Input: part model. Units: mm. Frame: model coordinates. Face numbers are marked on the shaded views. Round coordinates to 2 decimals unless told otherwise and drop trailing zeros. Loops run counter-clockwise (first coordinate to the right, second up) from the corner with the lowest first, then second, coordinate; pieces in that order, holes last. Notation, with made-up numbers: (15.5, -2.75) -> (65.5, -2.75) arc R28 ccw to (65.5, 16.25) -> close; hole circle Ø6 at (-27.75, 57). An arc over 180 degrees is marked (long way). One line per question, with ' | ' between items. Start each with the question number.
Q1. Material intervals for L1, parallel to Y at x = 30, z = 18; L2, parallel to Y at x = 28.25, z = 14.5; L3, parallel to Z at x = 38.75, y = -10.5, sorted ascending.
Q2. Contact query for flat-ended pins moving along their axis: P1, Ø5, axis at x = 39, y = 26, coming from the +Z side; P2, Ø3, axis at x = 28.5, y = 13.5, coming from the +Z side; P3, Ø8, axis at x = 28.5, z = 25.5, coming from the -Y side. Output: stop coordinate, or through.
Q3. Mould query, pull axis Y, two halves, no side actions, for the marked faces 1, 2 and 3. Classes: pulls with the +Y half, pulls with the -Y half, needs draft (parallel to the pull), parting line crosses it, or undercut.
Q4. Cut plane A-A on x = 46.75. Return loops of the section in (y, z).
Q5. Cut plane C-C on x = 36.75. Return loops of the section in (y, z).
Q6. Cut plane B-B on y = 0. Return loops of the section in (x, z).
from build123d import *

# Parameters (mm, degrees)
SKETCH001_W      = 178.926751
SKETCH001_H      = 164.552085
PAD_DEPTH        = 25
REVOLUTION_ANGLE = 180


with BuildPart() as pad:
    # Sketch001 → Pad (new body)
    with BuildSketch(Plane.YZ):
        with Locations((1.16814, -0.450252)):
            Rectangle(SKETCH001_W, SKETCH001_H)
    extrude(amount=PAD_DEPTH)


with BuildPart() as cut:
    # Sketch → Revolution (revolve)
    with BuildSketch(Plane.XY):
        Polygon((0, 25), (0, 75), (50, 25), align=None)
    revolve(axis=Axis((0, 0, 0), (1, 0, 0)), revolution_arc=REVOLUTION_ANGLE)

    # Cut: cut Pad
    add(pad.part, mode=Mode.SUBTRACT)


solid = cut.part
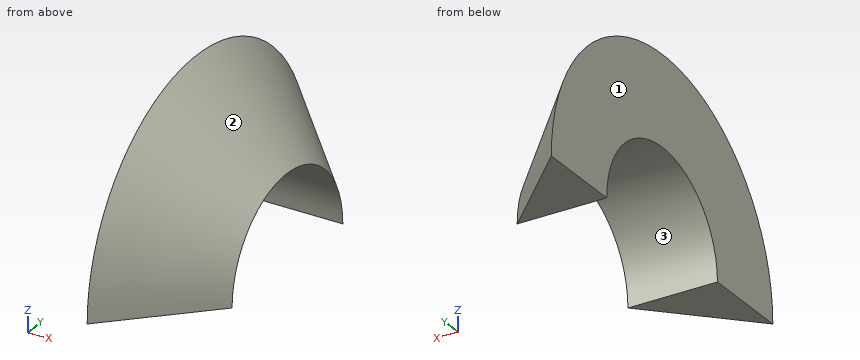
Results:
1) L1: -41.24 to -17.35, 17.35 to 41.24 | L2: -44.44 to -20.37, 20.37 to 44.44 | L3: 22.69 to 34.7
2) P1: z = 29.06 | P2: z = 46.12 | P3: y = -44.1
3) face 1: needs draft | face 2: parting line crosses it | face 3: undercut
4) outline: (-28.25, 0) -> (-25, 0) arc R25 cw to (25, 0) -> (28.25, 0) arc R28.25 ccw to start
5) outline: (-38.25, 0) -> (-25, 0) arc R25 cw to (25, 0) -> (38.25, 0) arc R38.25 ccw to start
6) outline: (25, 25) -> (50, 25) -> (25, 50) -> close
